Answer from the drawing. Dimensions are ordinates in mm from the lowest x, y and z of the part. Round coordinates to 2 decimals unless told otherwise and drop trailing zeros. Loops run counter-clockwise (first coordinate to the right, second up) from the corner with the lowest first, then second, coordinate; pieces in that order, holes last. Notation, with made-up numbers: M 2,27.5 L 17,27.5 A23 ccw 17,40.5 Z; hole C 61,-19 d5. An arc over 180 degrees is marked long. One line per item, written item: value.
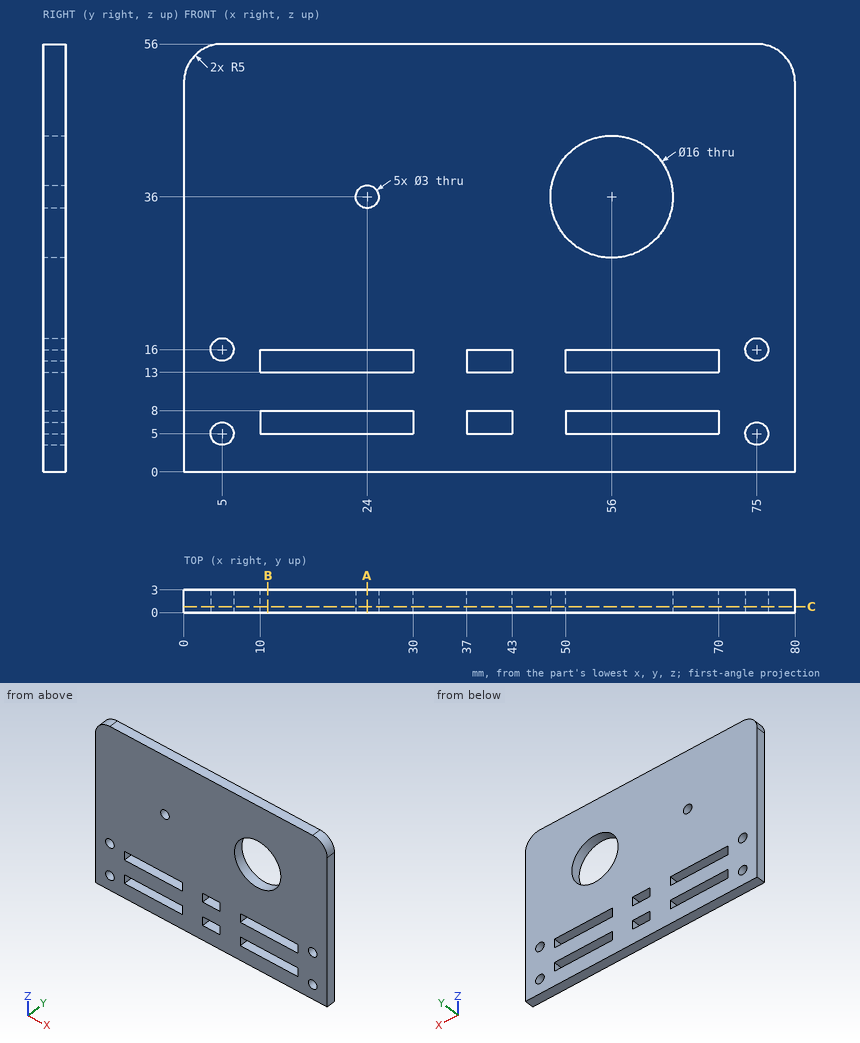
1) Find section C-C (y = 0.8). Give the number of separate pieces and of enclosed holes in the cut face, then the cut area to 3 significant figures.
Check values:
separate pieces: 1
enclosed holes: 12
area: 3,960 mm2
2) Find section B-B (x = 11). Give the vertices of the cut face in (y, z), then the cut area to 3 significant figures.
Check values:
outline: M 0,0 L 3,0 L 3,5 L 0,5 Z; M 0,8 L 3,8 L 3,13 L 0,13 Z; M 0,16 L 3,16 L 3,56 L 0,56 Z
area: 150 mm2
3) Find the intervals of material crossed by probe 1 along X at (y, z) = (2.1, 36); probe 2 along Z at (x, y) = (11, 1.4); probe 3 along X at (y, z) = (0.4, 7), in increasing order. Write a range as from..to.
Check values:
probe 1: 0..22.5, 25.5..48, 64..80
probe 2: 0..5, 8..13, 16..56
probe 3: 0..10, 30..37, 43..50, 70..80
4) Find section A-A (x = 24). Give the vertices of the cut face in (y, z).
Check values:
outline: M 0,0 L 3,0 L 3,5 L 0,5 Z; M 0,8 L 3,8 L 3,13 L 0,13 Z; M 0,16 L 3,16 L 3,34.5 L 0,34.5 Z; M 0,37.5 L 3,37.5 L 3,56 L 0,56 Z
5) This flat-tipped pin is pushed along its axis until it touches: pin 1 (3.5 mm diameter, centred on x = 5, z = 5, fed in from -Y). Where does it stop, or does it pass through?
Check values:
pin 1: y = 0
